Could you check a few things on this model? Use its own coordinates, in mm. A direction names the side the tool comes from. Round coordinates to 2 decimals unless told otherwise and drop trailing zeros. Loops run counter-clockwise (first coordinate to the right, second up) from the corner with the lowest first, then second, coordinate; pieces in that order, holes last.
from build123d import *

# Parameters (mm, degrees)
CROQUIS1_R                   = 44
CROQUIS1_R_2                 = 36.3
SALIENTE_EXTRUIR1_DEPTH      = 3
SALIENTE_EXTRUIR2_START      = 15
CROQUIS2_R                   = 44
CROQUIS2_R_2                 = 39
SALIENTE_EXTRUIR2_DEPTH      = 15
SALIENTE_EXTRUIR3_DEPTH      = 8.5
TALADRO_DE_MARGEN_PARA_M31_D = 3.4


with BuildPart() as part:
    # Croquis1 → Saliente-Extruir1 (new body)
    with BuildSketch(Plane.XY):
        Circle(CROQUIS1_R)
        Circle(CROQUIS1_R_2, mode=Mode.SUBTRACT)
    extrude(amount=SALIENTE_EXTRUIR1_DEPTH)

    # Croquis2 → Saliente-Extruir2 (add)
    with BuildSketch(Plane(origin=(0, 0, 0), x_dir=(-1, 0, 0), z_dir=(0, 0, -1)).offset(SALIENTE_EXTRUIR2_START)):
        Circle(CROQUIS2_R)
        Circle(CROQUIS2_R_2, mode=Mode.SUBTRACT)
    extrude(amount=-SALIENTE_EXTRUIR2_DEPTH)

    # Croquis3 → Saliente-Extruir3 (add)
    with BuildSketch(Plane(origin=(0, 0, -15), x_dir=(-1, 0, 0), z_dir=(0, 0, -1))):
        with BuildLine():
            Line((-29.439938859, 32.7), (-100, 32.7))
            Line((-100, 32.7), (-100, -32.7))
            Line((-100, -32.7), (-29.439938859, -32.7))
            ThreePointArc((-29.439938859, -32.7), (-44, 0), (-29.439938859, 32.7))
        make_face()
    extrude(amount=-SALIENTE_EXTRUIR3_DEPTH)

    # Taladro de margen para M31 (through all)
    with Locations(Plane(origin=(0, 0, -15), x_dir=(-1, 0, 0), z_dir=(0, 0, -1))):
        with Locations((-75, 0), (-90, 15), (-60, -15), (-60, 15), (-90, -15)):
            Hole(TALADRO_DE_MARGEN_PARA_M31_D / 2)


solid = part.part
Item 1: If we section it at B-B, the plane y = 0: Please give me the cut outline in (x, z), then the cut area to 3 significant figures.
Results list:
outline: (-44, -15) - (-39, -15) - (-39, 0) - (-36.3, 0) - (-36.3, 3) - (-44, 3) - close; (36.3, 0) - (39, 0) - (39, -15) - (73.3, -15) - (73.3, -6.5) - (44, -6.5) - (44, 3) - (36.3, 3) - close; (76.7, -15) - (100, -15) - (100, -6.5) - (76.7, -6.5) - close
area: 643 mm2
Item 2: If we section it at A-A, the plane x = 60: Please give me the cut outline in (y, z), then the cut area to 3 significant figures.
Results list:
outline: (-32.7, -15) - (-16.7, -15) - (-16.7, -6.5) - (-32.7, -6.5) - close; (-13.3, -15) - (13.3, -15) - (13.3, -6.5) - (-13.3, -6.5) - close; (16.7, -15) - (32.7, -15) - (32.7, -6.5) - (16.7, -6.5) - close
area: 498 mm2
Item 3: If I drill on line 1 along Y through (x, z) = (90, -11.5); line 2 along X through (y, z) = (-1, -7.5); line 3 along Y through (x, z) = (0, -9.5), over which ranges is the centre line in solid material (lowest first)?
Results list:
line 1: y = -32.7 to -16.7, -13.3 to 13.3, 16.7 to 32.7
line 2: x = -43.99 to -38.99, 38.99 to 73.63, 76.37 to 100
line 3: y = -44 to -39, 39 to 44
Item 4: If we section it at D-D, the plane z = -9.5: Please give me the cut outline in (x, y), then the cut area to 3 significant figures.
Results list:
outline: (29.44, -32.7) - (100, -32.7) - (100, 32.7) - (29.44, 32.7) arc R44 ccw (long way) to start; hole circle Ø78 at (0, 0); hole circle Ø3.4 at (60, -15); hole circle Ø3.4 at (60, 15); hole circle Ø3.4 at (75, 0); hole circle Ø3.4 at (90, -15); hole circle Ø3.4 at (90, 15)
area: 5,210 mm2
Item 5: Will these pins go through, and if not, where does the flat tip stop? pin 1 (4 mm diameter, centred on x = 54, z = -12.5, fed in from +Y); pin 2 (2 mm diameter, centred on x = 90, y = 15, fed in from -Z); pin 3 (1 mm diameter, centred on x = -13.5, z = -3.5, fed in from -Y); pin 4 (1.5 mm diameter, centred on x = -8.5, z = 0, fed in from -Y).
Results list:
pin 1: stops at y = 32.7
pin 2: passes through
pin 3: stops at y = -42.04
pin 4: stops at y = -43.31
Item 6: If we section it at C-C, the plane x = 0: Please give me the cut outline in (y, z), then the cut area to 3 significant figures.
Results list:
outline: (-44, -15) - (-39, -15) - (-39, 0) - (-36.3, 0) - (-36.3, 3) - (-44, 3) - close; (36.3, 0) - (39, 0) - (39, -15) - (44, -15) - (44, 3) - (36.3, 3) - close
area: 196 mm2
Item 7: We'd pull the mould along X, two halves only. Please class faces 1 (the flat face through (100, 0, -11)), 2 (the cylindrical face through (34.624, 10.904, 1.479)), 3 (the flat face through (6, 36, 3)): released by +X, released by -X, zero draft, split by the parting line, or undercut.
Results list:
face 1: released by +X
face 2: undercut
face 3: zero draft
Item 8: For faces 4 (the flat face through (64, 32.7, -11)), 5 (the flat face through (26, -26, 0)), 6 (the cylindrical face through (58.3, -14.93, -10.69)), 7 (the flat face through (65, -32.7, -11)), which set-ups out of +Z, -Z, +X, -X, +Y, -Y let a thin tool reach every point of the face, with its end or its side?
Results list:
face 4: +Z, -Z, +X, +Y
face 5: -Z
face 6: +Z, -Z
face 7: +Z, -Z, +X, -Y
